from build123d import *

# Parameters (mm, degrees)
SKETCH1_W           = 890
SKETCH1_H           = 850
BOSS_EXTRUDE1_DEPTH = 30
FILLET1_R           = 10
BOSS_EXTRUDE3_DEPTH = 70


with BuildPart() as part:
    # Sketch1 → Boss-Extrude1 (new body)
    with BuildSketch(Plane(origin=(0, 0, 0), x_dir=(0, 1, 0), z_dir=(0, 0, 1))):
        Rectangle(SKETCH1_W, SKETCH1_H)
    extrude(amount=BOSS_EXTRUDE1_DEPTH)

    # Fillet1
    fillet1_edges = [part.edges().sort_by_distance(p)[0] for p in [
        (-425, -445, 15),
        (-425, 445, 15),
        (425, 445, 15),
        (425, -445, 15),
    ]]
    fillet(fillet1_edges, radius=FILLET1_R)

    # Sketch3 → Boss-Extrude3 (add)
    with BuildSketch(Plane(origin=(0, 445, 0), x_dir=(-1, 0, 0), z_dir=(0, 1, 0))):
        Polygon((0, 0), (-150, 0), (-150, 30), (150, 30), (150, 0), align=None)
    extrude(amount=BOSS_EXTRUDE3_DEPTH)


solid = part.part
Verification items for the finished model (mm, model axes). A direction names the side the tool comes from. Give positions to 0.01 mm unless a question says otherwise; leave off trailing zeros. Loops run counter-clockwise (first coordinate to the right, second up) from the corner with the lowest first, then second, coordinate; pieces in that order, holes last.
1. Cross-section at B-B on x = 293.5. Record the cut outline in (y, z), and give its area (3 significant figures).
Derived:
outline: (-445, 0) - (445, 0) - (445, 30) - (-445, 30) - close
area: 26,700 mm2
2. Cross-section at A-A on z = 21.25. Record the cut outline in (x, y).
Derived:
outline: (-425, -435) arc R10 ccw to (-415, -445) - (415, -445) arc R10 ccw to (425, -435) - (425, 435) arc R10 ccw to (415, 445) - (150, 445) - (150, 515) - (-150, 515) - (-150, 445) - (-415, 445) arc R10 ccw to (-425, 435) - close
3. Tool access check on faces 1 (the flat face through (150, 480, 15)), 2 (the flat face through (-150, 480, 15)), 3 (the flat face through (-425, -6, 15)). Record the directions out of +Z, -Z, +X, -X, +Y, -Y that give a thin tool (end or side, any length) a straight path to the whole face; none if there is none.
Derived:
face 1: +Z, -Z, +X, +Y
face 2: +Z, -Z, -X, +Y
face 3: +Z, -Z, -X, +Y, -Y
4. Material ranges on probe 1 along Y at (x, z) = (-342, 23), recorded low to high.
Derived:
probe 1: y = -445 to 445
5. Go/stop test with a flat-tipped pin: P1, Ø6, axis at x = 252.5, z = 11, coming from the +Y side. Record where the tip stops, or that it passes through.
Derived:
P1: stops at y = 445
